```python
from build123d import *

# Parameters (mm, degrees)
SKETCH_1_W                  = 86
SKETCH_1_H                  = 43
EXTRUDE_1_DEPTH             = 39.5
EXTRUDE_2_DEPTH             = 5
SKETCH_3_W                  = 80.6
SKETCH_3_H                  = 40.2
CUT_EXTRUDE_1_DEPTH         = 43.6
HOLE_WIZARD_8_3_8_3_1_D     = 8.3
HOLE_WIZARD_8_3_8_3_1_DEPTH = 3.2
FILLET_1_R                  = 3
EXTRUDE_START               = -4
SKETCH_6_R                  = 4.15
EXTRUDE_3_DEPTH             = 4
EXTRUDE_4_DEPTH             = 42
SKETCH_10_W                 = 2.2
SKETCH_10_H                 = 43
EXTRUDE_5_DEPTH             = 42
FILLET_2_R                  = 2


with BuildPart() as part:
    # Эскиз1 → Бобышка-Вытянуть1 (new body)
    with BuildSketch(Plane.XY.offset(22.25)):
        with Locations((47, 0)):
            Rectangle(SKETCH_1_W, SKETCH_1_H)
    extrude(amount=-EXTRUDE_1_DEPTH)

    # Эскиз2 → Бобышка-Вытянуть2 (add)
    with BuildSketch(Plane(origin=(0, 0, -17.25), x_dir=(-1, 0, 0), z_dir=(0, 0, -1))):
        with BuildLine():
            Line((-90, -21.5), (-90, -16.5))
            ThreePointArc((-90, -16.5), (-104, 0), (-90, 16.5))
            Line((-90, 16.5), (-90, 21.5))
            Line((-90, 21.5), (-4, 21.5))
            Line((-4, 21.5), (-4, -21.5))
            Line((-4, -21.5), (-90, -21.5))
        make_face()
        with BuildLine():
            Line((-90, -12.428366172), (-90, 12.428366172))
            ThreePointArc((-90, 12.428366172), (-100, 0), (-90, -12.428366172))
        make_face(mode=Mode.SUBTRACT)
    extrude(amount=EXTRUDE_2_DEPTH)

    # Эскиз3 → Вырез-Вытянуть1 (cut)
    with BuildSketch(Plane.XY.offset(22.25)):
        with Locations((48.3, 0)):
            Rectangle(SKETCH_3_W, SKETCH_3_H)
    extrude(amount=-CUT_EXTRUDE_1_DEPTH, mode=Mode.SUBTRACT)

    # Диаметр отверстия Ø8.3 (8.3)1
    with Locations(Plane.ZY.offset(-4)):
        with Locations((0, 0)):
            Hole(HOLE_WIZARD_8_3_8_3_1_D / 2, depth=HOLE_WIZARD_8_3_8_3_1_DEPTH)

    # Скругление1
    fillet_1_edges = [part.edges().sort_by_distance(p)[0] for p in [
        (4, -21.5, 0),
        (4, 21.5, 0),
    ]]
    fillet(fillet_1_edges, radius=FILLET_1_R)

    # Эскиз6 → Бобышка-Вытянуть3 (add)
    with BuildSketch(Plane.ZY.offset(-4).offset(EXTRUDE_START)):
        Circle(SKETCH_6_R)
    extrude(amount=EXTRUDE_3_DEPTH)

    # Эскиз7 → Бобышка-Вытянуть4 (add)
    with BuildSketch(Plane(origin=(0, 0, -22.25), x_dir=(-1, 0, 0), z_dir=(0, 0, -1))):
        Polygon((-90, -1.1), (-90, 1.1), (-4, 1.1), (-4, 0), (-4, -1.1), align=None)
    extrude(amount=-EXTRUDE_4_DEPTH)

    # Эскиз10 → Бобышка-Вытянуть5 (add)
    with BuildSketch(Plane(origin=(0, 0, -22.25), x_dir=(-1, 0, 0), z_dir=(0, 0, -1))):
        with Locations((-47.4, 0)):
            Rectangle(SKETCH_10_W, SKETCH_10_H)
    extrude(amount=-EXTRUDE_5_DEPTH)

    # Скругление2
    fillet_2_edges = [part.edges().sort_by_distance(p)[0] for p in [
        (27.15, 1.1, -21.35),
        (48.5, 1.1, -0.8),
        (46.3, 1.1, -0.8),
        (68.55, -1.1, -21.35),
        (27.15, 20.1, -21.35),
        (68.55, -20.1, -21.35),
        (46.3, -1.1, -0.8),
        (46.3, -10.6, -21.35),
        (46.3, 10.6, -21.35),
        (48.5, -10.6, -21.35),
        (48.5, -1.1, -0.8),
        (48.5, 10.6, -21.35),
        (46.3, -20.1, -0.8),
        (46.3, 20.1, -0.8),
        (48.5, -20.1, -0.8),
        (48.5, 20.1, -0.8),
        (27.15, -20.1, -21.35),
        (88.6, -20.1, 0.45),
        (8, 10.6, -21.35),
        (8, -20.1, 0.45),
        (68.55, 20.1, -21.35),
        (8, 20.1, 0.45),
        (88.6, -10.6, -21.35),
        (88.6, 20.1, 0.45),
        (88.6, 10.6, -21.35),
        (8, -10.6, -21.35),
        (68.55, 1.1, -21.35),
        (27.15, -1.1, -21.35),
        (8, -1.1, -0.8),
        (88.6, -1.1, -0.8),
        (8, 1.1, -0.8),
        (88.6, 1.1, -0.8),
    ]]
    fillet(fillet_2_edges, radius=FILLET_2_R)


solid = part.part
```
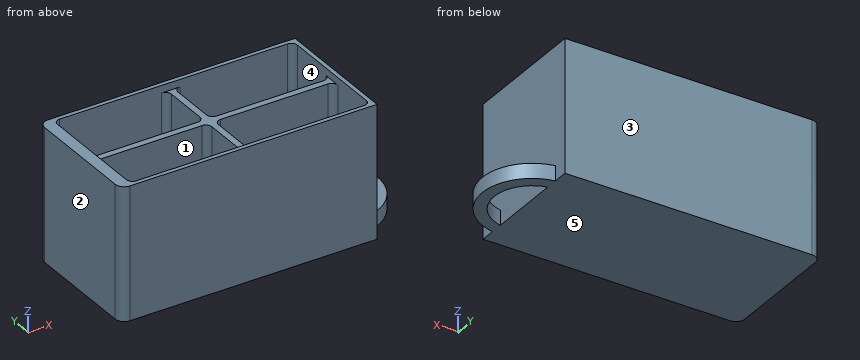
Verification items for the finished model (mm, model axes). Face numbers are marked on the shaded views. A direction names the side the tool comes from. Coordinates: 2 decimals unless noted, no trailing zeros. Loops run counter-clockwise (first coordinate to the right, second up) from the corner with the lowest first, then second, coordinate; pieces in that order, holes last. Notation, with made-up numbers: (18.5, -9) -> (51.5, -9) arc R13 cw to (51.5, 1) -> close; hole circle Ø1 at (-36, -30.75). An arc over 180 degrees is marked (long way). Answer in a Markdown table with one row per item.
1) Depth check by flat-ended pin: P1, Ø1, axis at y = 10.5, z = 9.5, coming from the +X side; P2, Ø1, axis at x = 18, y = -15, coming from the +Z side; P3, Ø11, axis at x = 94, y = -0.5, coming from the +Z side. Enter the tip coordinate at first touch or a pass-through.
The answers:
| item | result |
|---|---|
| P1 | stops at x = 90 |
| P2 | stops at z = -21.35 |
| P3 | stops at z = 22.25 |
2) Access from +Z, -Z, +X, -X, +Y, -Y to the whole of each face (thin tool, end or side, straight path). Record for the marked faces 1 and 2.
The answers:
| item | result |
|---|---|
| face 1 | +Z |
| face 2 | +Z, -Z, -X, +Y, -Y |
3) Scan lines: line 1 along Y through (x, z) = (67, 2); line 2 along X through (y, z) = (-3, 5.5); line 3 along Y through (x, z) = (45, 3). Record each from-to range of solid material in increasing order. Write a range as from..to.
The answers:
| item | result |
|---|---|
| line 1 | y = -21.5..-20.1, -1.1..1.1, 20.1..21.5 |
| line 2 | x = 4..8, 46.3..48.5, 88.6..90 |
| line 3 | y = -21.5..-19.97, -1.23..1.23, 19.97..21.5 |
4) Section check C-C (x = 30). Record the cut outline in (y, z).
The answers:
| item | result |
|---|---|
| outline | (-21.5, -22.25) -> (21.5, -22.25) -> (21.5, 22.25) -> (20.1, 22.25) -> (20.1, -19.35) arc R2 cw to (18.1, -21.35) -> (3.1, -21.35) arc R2 cw to (1.1, -19.35) -> (1.1, 19.75) -> (-1.1, 19.75) -> (-1.1, -19.35) arc R2 cw to (-3.1, -21.35) -> (-18.1, -21.35) arc R2 cw to (-20.1, -19.35) -> (-20.1, 22.25) -> (-21.5, 22.25) -> close |
5) Draft check along Y on the marked faces 3, 4 and 5. Enter one of: released by +Y, released by -Y, zero draft, split by the parting line, or undercut.
The answers:
| item | result |
|---|---|
| face 3 | released by +Y |
| face 4 | undercut |
| face 5 | zero draft |
6) Section check A-A (y = 6). Record the cut outline in (x, z).
The answers:
| item | result |
|---|---|
| outline | (4, -22.25) -> (90, -22.25) -> (90, 22.25) -> (88.6, 22.25) -> (88.6, -19.35) arc R2 cw to (86.6, -21.35) -> (50.5, -21.35) arc R2 cw to (48.5, -19.35) -> (48.5, 19.75) -> (46.3, 19.75) -> (46.3, -19.35) arc R2 cw to (44.3, -21.35) -> (10, -21.35) arc R2 cw to (8, -19.35) -> (8, 22.25) -> (4, 22.25) -> close; (98.5, -22.25) -> (102.89, -22.25) -> (102.89, -17.25) -> (98.5, -17.25) -> close |
7) Section check B-B (x = 91). Record the cut outline in (y, z), and give its area (3 significant figures).
The answers:
| item | result |
|---|---|
| outline | (-16.3, -22.25) -> (-12.17, -22.25) -> (-12.17, -17.25) -> (-16.3, -17.25) -> close; (12.17, -22.25) -> (16.3, -22.25) -> (16.3, -17.25) -> (12.17, -17.25) -> close |
| area | 41.4 mm2 |
8) Section check D-D (y = -14). Record the cut outline in (x, z).
The answers:
| item | result |
|---|---|
| outline | (4, -22.25) -> (96.42, -22.25) -> (96.42, -17.25) -> (90, -17.25) -> (90, 22.25) -> (88.6, 22.25) -> (88.6, -19.35) arc R2 cw to (86.6, -21.35) -> (50.5, -21.35) arc R2 cw to (48.5, -19.35) -> (48.5, 19.75) -> (46.3, 19.75) -> (46.3, -19.35) arc R2 cw to (44.3, -21.35) -> (10, -21.35) arc R2 cw to (8, -19.35) -> (8, 22.25) -> (4, 22.25) -> close |
